Input: part model. Units: mm. Frame: model coordinates. Face numbers are marked on the shaded views. Coordinates: 2 decimals unless noted, no trailing zeros. Order: outer loops, then holes, each group sorted by start corner. A loop starts at its lowest first (then second) coordinate and runs counter-clockwise, first axis right, second up. Notation, with made-up numbers: (3, 68.5) - (50, 68.5) arc R19 cw to (50, 93.5) - close; hole circle Ø1 at (46, -9.75). An arc over 180 degrees is marked (long way). Use a Markdown table: item, result. Add a question column.
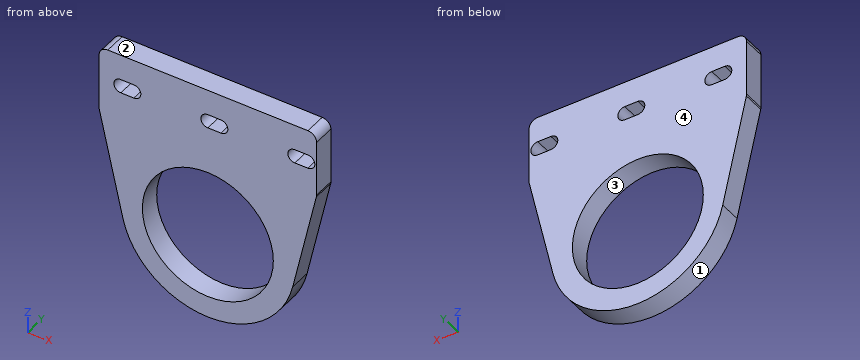
from build123d import *

# Parameters (mm, degrees)
SKETCH_1_R          = 20
SKETCH_1_R_2        = 6.5
SKETCH_1_R_3        = 1.6
EXTRUDE_1_DEPTH     = 5
SKETCH_2_W          = 50
SKETCH_2_H          = 15
SKETCH_2_R          = 1.6
EXTRUDE_2_DEPTH     = 5
EXTRUDE_START       = -5
EXTRUDE_4_DEPTH     = 5
SKETCH_5_R          = 3.5
CUT_EXTRUDE_1_DEPTH = 3
FILLET_1_R          = 2
SKETCH_6_R          = 15.05
CUT_EXTRUDE_2_DEPTH = 44.301270189
CUT_EXTRUDE_3_DEPTH = 44.301270189


with BuildPart() as part:
    # Sketch 1 → Extrude 1 (new body)
    with BuildSketch(Plane(origin=(0, 0, 0), x_dir=(1, 0, 0), z_dir=(0, 1, 0))):
        with Locations(Location((0, 0, 0), (0, 0, 270))):
            Circle(SKETCH_1_R)
        with Locations(Location((0, 0, 0), (0, 0, 270))):
            Circle(SKETCH_1_R_2, mode=Mode.SUBTRACT)
        with Locations(Location((0, 9.5, 0), (0, 0, 270))):
            Circle(SKETCH_1_R_3, mode=Mode.SUBTRACT)
        with Locations(Location((8.227241336, -4.75, 0), (0, 0, 270))):
            Circle(SKETCH_1_R_3, mode=Mode.SUBTRACT)
        with Locations(Location((-8.227241336, -4.75, 0), (0, 0, 270))):
            Circle(SKETCH_1_R_3, mode=Mode.SUBTRACT)
    extrude(amount=EXTRUDE_1_DEPTH)



with BuildPart() as body_2:
    # Sketch 2 → Extrude 2 (new body)
    with BuildSketch(Plane(origin=(0, 5, 0), x_dir=(1, 0, 0), z_dir=(0, 1, 0))):
        with Locations((0, -27.5)):
            Rectangle(SKETCH_2_W, SKETCH_2_H)
        with Locations(Location((-20, -27.5, 0), (0, 0, 270))):
            Circle(SKETCH_2_R, mode=Mode.SUBTRACT)
        with Locations(Location((20, -27.5, 0), (0, 0, 270))):
            Circle(SKETCH_2_R, mode=Mode.SUBTRACT)
        with Locations(Location((0, -27.5, 0), (0, 0, 270))):
            Circle(SKETCH_2_R, mode=Mode.SUBTRACT)
    extrude(amount=-EXTRUDE_2_DEPTH)


with BuildPart() as part_1:
    add(part.part)

    add(body_2.part)  # Extrude 4 merges body 2
    # Sketch 4 → Extrude 4 (add)
    with BuildSketch(Plane(origin=(0, 5, 0), x_dir=(1, 0, 0), z_dir=(0, 1, 0)).offset(EXTRUDE_START)):
        with BuildLine():
            Line((-19.512195122, 4.390243902), (-25, -20))
            Line((-25, -20), (0, -20))
            ThreePointArc((0, -20), (-15.617376189, -12.493900951), (-19.512195122, 4.390243902))
        make_face()
        with BuildLine():
            ThreePointArc((20, 0), (14.142135624, -14.142135624), (0, -20))
            Line((0, -20), (25, -20))
            Line((25, -20), (19.512195122, 4.390243902))
            ThreePointArc((19.512195122, 4.390243902), (19.877674693, 2.208630521), (20, 0))
        make_face()
    extrude(amount=EXTRUDE_4_DEPTH)

    # Sketch 5 → Cut-Extrude 1 (cut)
    with BuildSketch(Plane(origin=(0, 5, 0), x_dir=(1, 0, 0), z_dir=(0, 1, 0))):
        with Locations((-8.227241336, -4.75)):
            Circle(SKETCH_5_R)
        with Locations((8.227241336, -4.75)):
            Circle(SKETCH_5_R)
        with Locations((0, 9.5)):
            Circle(SKETCH_5_R)
    extrude(amount=-CUT_EXTRUDE_1_DEPTH, mode=Mode.SUBTRACT)

    # Fillet 1
    fillet_1_edges = [part_1.edges().sort_by_distance(p)[0] for p in [
        (-25, 2.5, 20),
        (25, 2.5, 20),
        (25, 2.5, 35),
        (-25, 2.5, 35),
    ]]
    fillet(fillet_1_edges, radius=FILLET_1_R)

    # Sketch 6 → Cut-Extrude 2 (cut, through all)
    with BuildSketch(Plane(origin=(0, 5, 0), x_dir=(1, 0, 0), z_dir=(0, 1, 0))):
        with Locations(Location((0, 0, 0), (0, 0, 270))):
            Circle(SKETCH_6_R)
    extrude(amount=-CUT_EXTRUDE_2_DEPTH, mode=Mode.SUBTRACT)

    # Sketch 7 → Cut-Extrude 3 (cut, through all)
    with BuildSketch(Plane(origin=(0, 5, 0), x_dir=(1, 0, 0), z_dir=(0, 1, 0))):
        with BuildLine():
            Line((-20, -25.9), (-17, -25.9))
            ThreePointArc((-17, -25.9), (-15.4, -27.5), (-17, -29.1))
            Line((-17, -29.1), (-20, -29.1))
            ThreePointArc((-20, -29.1), (-21.6, -27.5), (-20, -25.9))
        make_face()
        with BuildLine():
            Line((0, -25.9), (3, -25.9))
            ThreePointArc((3, -25.9), (4.6, -27.5), (3, -29.1))
            Line((3, -29.1), (0, -29.1))
            ThreePointArc((0, -29.1), (-1.6, -27.5), (0, -25.9))
        make_face()
        with BuildLine():
            Line((20, -25.9), (23, -25.9))
            ThreePointArc((23, -25.9), (24.6, -27.5), (23, -29.1))
            Line((23, -29.1), (20, -29.1))
            ThreePointArc((20, -29.1), (18.4, -27.5), (20, -25.9))
        make_face()
    extrude(amount=-CUT_EXTRUDE_3_DEPTH, mode=Mode.SUBTRACT)


solid = part_1.part
1) Contact query for flat-ended pins moving along their axis: P1, Ø2, axis at x = -5.5, y = 3.5, coming from the -Z side; P2, Ø1, axis at x = 19, y = 3, coming from the -Z side; P3, Ø1.5, axis at y = 0.5, z = -10, coming from the +X side. Output: stop coordinate, or through.
2) Material intervals for L1, parallel to X at y = 3.95, z = 0; L2, parallel to Z at x = -12.5, y = 1.7; L3, parallel to X at y = 2.7, z = 28, sorted ascending.
3) Cut plane A-A (z = 0). Return the cut outline in (x, y).
4) Cut plane C-C (x = -18). Return the cut outline in (y, z), and give its area (3 significant figures).
5) Pull-direction query (Z, two-part tool) for the marked faces 1, 2, 3 and 4; classes: pulls with the +Z half, pulls with the -Z half, needs draft (parallel to the pull), parting line crosses it, or undercut.
6) Cut plane B-B (y = 1.55). Return the cut outline in (x, z), and give its area (3 significant figures).
Computed:
| question | item | result |
|---|---|---|
| 1 | P1 | stops at z = -19.49 |
| 1 | P2 | stops at z = -7.6 |
| 1 | P3 | stops at x = 17.73 |
| 2 | L1 | x = -20.5 to -15.05, 15.05 to 20.5 |
| 2 | L2 | z = -15.61 to -8.38, 8.38 to 35 |
| 2 | L3 | x = -25 to -21.52, -15.48 to -1.52, 4.52 to 18.48, 24.52 to 25 |
| 3 | outline | (-20.5, 0) - (-15.05, 0) - (-15.05, 5) - (-20.5, 5) - close; (15.05, 0) - (20.5, 0) - (20.5, 5) - (15.05, 5) - close |
| 4 | outline | (0, -8.72) - (5, -8.72) - (5, 25.9) - (0, 25.9) - close; (0, 29.1) - (5, 29.1) - (5, 35) - (0, 35) - close |
| 4 | area | 203 mm2 |
| 5 | face 1 | pulls with the -Z half |
| 5 | face 2 | pulls with the +Z half |
| 5 | face 3 | undercut |
| 5 | face 4 | needs draft |
| 6 | outline | (-25, 20.22) arc R2 ccw to (-24.95, 19.78) - (-19.51, -4.39) arc R20 ccw to (19.51, -4.39) - (24.95, 19.78) arc R2 ccw to (25, 20.22) - (25, 33) arc R2 ccw to (23, 35) - (-23, 35) arc R2 ccw to (-25, 33) - close; hole (-20, 25.9) - (-17, 25.9) arc R1.6 ccw to (-17, 29.1) - (-20, 29.1) arc R1.6 ccw to start; hole circle Ø30.1 at (0, 0); hole (0, 25.9) - (3, 25.9) arc R1.6 ccw to (3, 29.1) - (0, 29.1) arc R1.6 ccw to start; hole (20, 25.9) - (23, 25.9) arc R1.6 ccw to (23, 29.1) - (20, 29.1) arc R1.6 ccw to start |
| 6 | area | 1,520 mm2 |
